from build123d import *

# Parameters (mm, degrees)
MASTER_SKETCH_W           = 688.4416
MASTER_SKETCH_H           = 498.348
BOSS_EXTRUDE1_DEPTH       = 3.175
SKETCH1_W                 = 28.575
SKETCH1_H                 = 498.348
BOSS_EXTRUDE2_DEPTH       = 3.175
M6_CLEARANCE_HOLE1_D      = 6.6
SKETCH5_W                 = 2.286
SKETCH5_H                 = 69.85
CUT_EXTRUDE1_DEPTH        = 449.413281916
LPATTERN1_COUNT           = 5
LPATTERN1_PITCH           = 98.8568
SKETCH6_W                 = 254
SKETCH6_H                 = 3.175
CUT_EXTRUDE2_DEPTH        = 449.413281916
SKETCH7_W                 = 254
SKETCH7_H                 = 2.286
CUT_EXTRUDE3_DEPTH        = 449.413281916
LPATTERN2_COUNT           = 4
LPATTERN2_PITCH           = 98.8568
SKETCH8_R                 = 5
CUT_EXTRUDE4_DEPTH        = 449.413281916
LPATTERN3_COUNT           = 2
LPATTERN3_PITCH           = 197.7136
LPATTERN3_COPY_1_SKETCH_R = 5
LPATTERN3_COPY_1_DEPTH    = 449.413281916
SKETCH9_R                 = 5
CUT_EXTRUDE5_DEPTH        = 449.413281916
LPATTERN4_COUNT           = 4
LPATTERN4_PITCH           = 98.8568
LPATTERN4_COPY_1_SKETCH_R = 5
LPATTERN4_COPY_1_DEPTH    = 449.413281916
LPATTERN4_COPY_2_SKETCH_R = 5
LPATTERN4_COPY_2_DEPTH    = 449.413281916


with BuildPart() as part:
    # Master Sketch → Boss-Extrude1 (new body)
    with BuildSketch(Plane.XY):
        Rectangle(MASTER_SKETCH_W, MASTER_SKETCH_H)
    extrude(amount=BOSS_EXTRUDE1_DEPTH)

    # Sketch1 → Boss-Extrude2 (add)
    with BuildSketch(Plane.XY.offset(3.175)):
        with Locations((-358.5083, 0)):
            Rectangle(SKETCH1_W, SKETCH1_H)
    boss_extrude2 = extrude(amount=-BOSS_EXTRUDE2_DEPTH)

    # M6 Clearance Hole1 (through all)
    with Locations(Plane.XY.offset(3.175)):
        with Locations((-358.5083, -197.612), (-358.5083, -98.806), (-358.5083, 0), (-358.5083, 98.806), (-358.5083, 197.612)):
            m6_clearance_hole1 = Hole(M6_CLEARANCE_HOLE1_D / 2)

    # Mirror1: Boss-Extrude2, M6 Clearance Hole1 across plane
    add(boss_extrude2.mirror(Plane(origin=(0, 0, 0), x_dir=(0, 0, 1), z_dir=(1, 0, 0))))
    add(m6_clearance_hole1.mirror(Plane(origin=(0, 0, 0), x_dir=(0, 0, 1), z_dir=(1, 0, 0))), mode=Mode.SUBTRACT)

    # Sketch5 → Cut-Extrude1 (cut, through all)
    with BuildSketch(Plane.XY.offset(3.175)):
        with Locations((26.543, 197.7136)):
            Rectangle(SKETCH5_W, SKETCH5_H)
        with Locations((-26.543, 197.7136)):
            Rectangle(SKETCH5_W, SKETCH5_H)
    cut_extrude1 = extrude(amount=-CUT_EXTRUDE1_DEPTH, mode=Mode.SUBTRACT)

    # LPattern1: Cut-Extrude1 ×5
    with Locations(*[(0, -i * LPATTERN1_PITCH, 0) for i in range(1, LPATTERN1_COUNT)]):
        add(cut_extrude1, mode=Mode.SUBTRACT)

    # Sketch6 → Cut-Extrude2 (cut, through all)
    with BuildSketch(Plane.XY.offset(3.175)):
        with Locations((-184.3659, 247.5865)):
            Rectangle(SKETCH6_W, SKETCH6_H)
        with Locations((184.3659, 247.5865)):
            Rectangle(SKETCH6_W, SKETCH6_H)
    cut_extrude2 = extrude(amount=-CUT_EXTRUDE2_DEPTH, mode=Mode.SUBTRACT)

    # Mirror2: Cut-Extrude2 across plane
    add(cut_extrude2.mirror(Plane.ZX), mode=Mode.SUBTRACT)

    # Sketch7 → Cut-Extrude3 (cut, through all)
    with BuildSketch(Plane.XY.offset(3.175)):
        with Locations((-184.3659, 148.2852)):
            Rectangle(SKETCH7_W, SKETCH7_H)
        with Locations((184.3659, 148.2852)):
            Rectangle(SKETCH7_W, SKETCH7_H)
    cut_extrude3 = extrude(amount=-CUT_EXTRUDE3_DEPTH, mode=Mode.SUBTRACT)

    # LPattern2: Cut-Extrude3 ×4
    with Locations(*[(0, -i * LPATTERN2_PITCH, 0) for i in range(1, LPATTERN2_COUNT)]):
        add(cut_extrude3, mode=Mode.SUBTRACT)

    # Sketch8 → Cut-Extrude4 (cut, through all)
    with BuildSketch(Plane(origin=(0, 0, 0), x_dir=(-1, 0, 0), z_dir=(0, 0, -1))):
        with Locations((8.255, -155.591933333)):
            Circle(SKETCH8_R)
        with Locations((19.685, -155.591933333)):
            Circle(SKETCH8_R)
        with Locations((13.97, -167.021933333)):
            Circle(SKETCH8_R)
    cut_extrude4 = extrude(amount=-CUT_EXTRUDE4_DEPTH, mode=Mode.SUBTRACT)

    # Mirror3: Cut-Extrude4 across plane
    add(cut_extrude4.mirror(Plane(origin=(0, 0, 0), x_dir=(0, 0, 1), z_dir=(1, 0, 0))), mode=Mode.SUBTRACT)

    # LPattern3: Cut-Extrude4 ×2
    with Locations(*[(0, i * LPATTERN3_PITCH, 0) for i in range(1, LPATTERN3_COUNT)]):
        add(cut_extrude4, mode=Mode.SUBTRACT)

    # LPattern3 copy 1 sketch → LPattern3 copy 1 (cut, through all)
    with BuildSketch(Plane(origin=(0, 197.7136, 0), x_dir=(1, 0, 0), z_dir=(0, 0, -1))):
        with Locations((8.255, 155.591933333)):
            Circle(LPATTERN3_COPY_1_SKETCH_R)
        with Locations((19.685, 155.591933333)):
            Circle(LPATTERN3_COPY_1_SKETCH_R)
        with Locations((13.97, 167.021933333)):
            Circle(LPATTERN3_COPY_1_SKETCH_R)
    extrude(amount=-LPATTERN3_COPY_1_DEPTH, mode=Mode.SUBTRACT)

    # Sketch9 → Cut-Extrude5 (cut, through all)
    with BuildSketch(Plane(origin=(0, 0, 0), x_dir=(-1, 0, 0), z_dir=(0, 0, -1))):
        with Locations((8.255, -140.978466667)):
            Circle(SKETCH9_R)
        with Locations((13.97, -129.548466667)):
            Circle(SKETCH9_R)
        with Locations((19.685, -140.978466667)):
            Circle(SKETCH9_R)
    cut_extrude5 = extrude(amount=-CUT_EXTRUDE5_DEPTH, mode=Mode.SUBTRACT)

    # Mirror4: Cut-Extrude5 across plane
    add(cut_extrude5.mirror(Plane(origin=(0, 0, 0), x_dir=(0, 0, 1), z_dir=(1, 0, 0))), mode=Mode.SUBTRACT)

    # LPattern4: Cut-Extrude5 ×4, 1 skipped
    with Locations(*[(0, i * LPATTERN4_PITCH, 0) for i in range(1, LPATTERN4_COUNT) if i not in (1,)]):
        add(cut_extrude5, mode=Mode.SUBTRACT)

    # LPattern4 copy 1 sketch → LPattern4 copy 1 (cut, through all)
    with BuildSketch(Plane(origin=(0, 197.7136, 0), x_dir=(1, 0, 0), z_dir=(0, 0, -1))):
        with Locations((8.255, 140.978466667)):
            Circle(LPATTERN4_COPY_1_SKETCH_R)
        with Locations((13.97, 129.548466667)):
            Circle(LPATTERN4_COPY_1_SKETCH_R)
        with Locations((19.685, 140.978466667)):
            Circle(LPATTERN4_COPY_1_SKETCH_R)
    extrude(amount=-LPATTERN4_COPY_1_DEPTH, mode=Mode.SUBTRACT)

    # LPattern4 copy 2 sketch → LPattern4 copy 2 (cut, through all)
    with BuildSketch(Plane(origin=(0, 296.5704, 0), x_dir=(1, 0, 0), z_dir=(0, 0, -1))):
        with Locations((8.255, 140.978466667)):
            Circle(LPATTERN4_COPY_2_SKETCH_R)
        with Locations((13.97, 129.548466667)):
            Circle(LPATTERN4_COPY_2_SKETCH_R)
        with Locations((19.685, 140.978466667)):
            Circle(LPATTERN4_COPY_2_SKETCH_R)
    extrude(amount=-LPATTERN4_COPY_2_DEPTH, mode=Mode.SUBTRACT)


solid = part.part
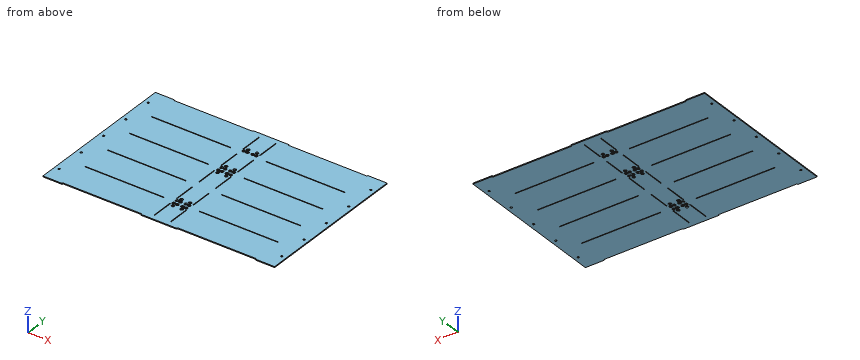
Verification items for the finished model (mm, model axes). Coordinates: 2 decimals unless noted, no trailing zeros. Write each loop counter-clockwise with the first axis right and the second up, starting at its lowest first coordinate (ties: lowest second). Pieces come first, ordered by that corner, then holes. Notation, with made-up numbers: (87.25, 77.5) -> (114.25, 77.5) arc R20 cw to (114.25, 107.5) -> close; hole circle Ø9 at (65, 43). An arc over 180 degrees is marked (long way). One line per item, written item: value. Start each with the question number.
Q1. Go/stop test with flat-tipped pins: P1, Ø1.5, axis at x = -58.5, z = 1, coming from the +Y side; P2, Ø8, axis at x = 19.68, y = 42.12, coming from the -Z side. Record where each tip stops, or that it passes through.
Q2. Cross-section at B-B on z = 1.1. State how many separate pieces and enclosed holes the cut face has, and give its area (3 significant figures).
Q3. Cross-section at A-A on x = 153.5. Enter the section's corners in (y, z) (3 decimals), and give its area (3 significant figures).
Q4. Thickness scan on L1, parallel to X at y = 173.5, z = 2.7; L2, parallel to Y at x = 68.5, z = 2.7; L3, parallel to X at y = -168, z = 1.4. Record the ranges inside material, lowest first. Write a range as from..to.
Checked values:
1. P1: stops at y = 246
1. P2: passes through
2. separate pieces: 1
2. enclosed holes: 58
2. area: 359,000 mm²
3. outline: (-245.999, 0) -> (-149.428, 0) -> (-149.428, 3.175) -> (-245.999, 3.175) -> close; (-147.142, 0) -> (-50.571, 0) -> (-50.571, 3.175) -> (-147.142, 3.175) -> close; (-48.285, 0) -> (48.285, 0) -> (48.285, 3.175) -> (-48.285, 3.175) -> close; (50.571, 0) -> (147.142, 0) -> (147.142, 3.175) -> (50.571, 3.175) -> close; (149.428, 0) -> (245.999, 0) -> (245.999, 3.175) -> (149.428, 3.175) -> close
3. area: 1,530 mm²
4. L1: x = -372.8..-27.69, -25.4..25.4, 27.69..372.8
4. L2: y = -246..-149.43, -147.14..-50.57, -48.29..48.29, 50.57..147.14, 149.43..246
4. L3: x = -372.8..-27.69, -25.4..-18.87, -9.07..9.07, 18.87..25.4, 27.69..372.8
